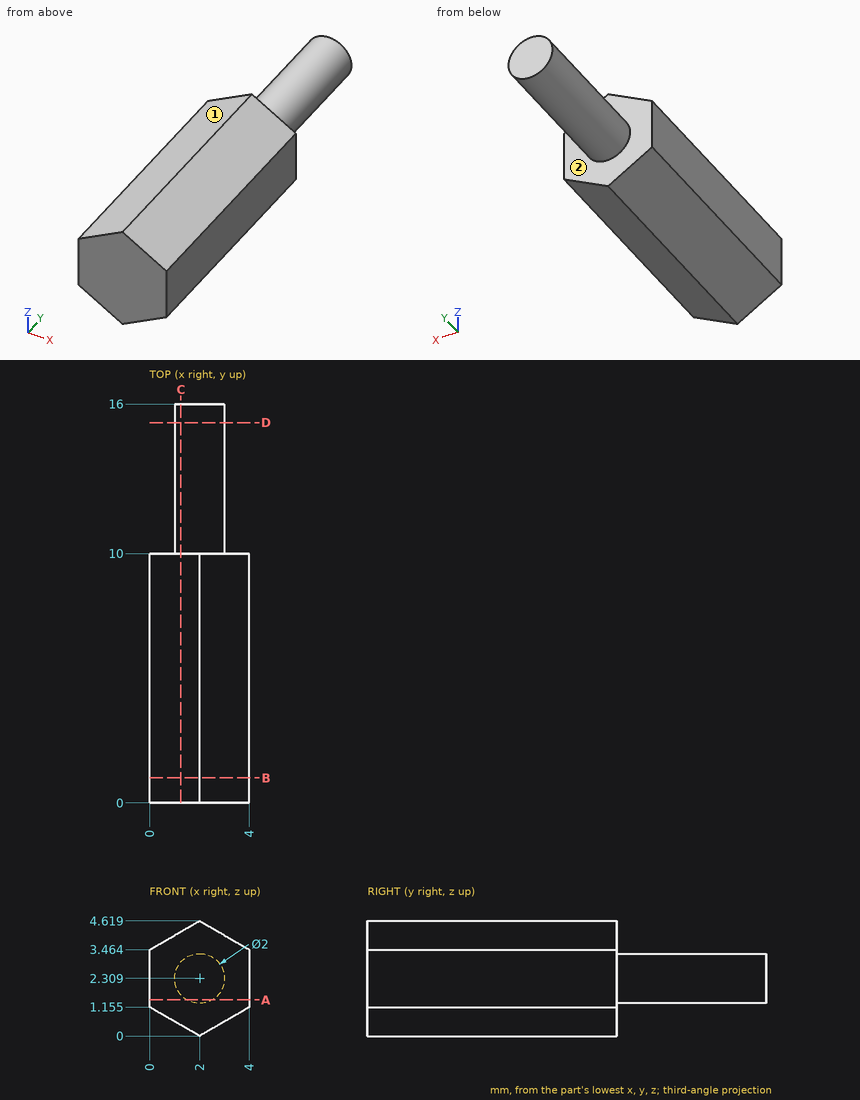
Geometry check sheet. Reference: drawing and pictorial views, mm from the part's lowest x, y, z. A direction names the side the tool comes from. Give positions to 0.01 mm unless a question says otherwise; leave off trailing zeros. Order: outer loops, then holes, each group sorted by start corner. A loop starts at its lowest first (then second) coordinate and runs counter-clockwise, first axis right, second up. Notation, with made-up numbers: M 73.5,46 L 102.5,46 A20 cw 102.5,68 Z; hole C -24,5.25 d8. An arc over 180 degrees is marked long. Answer in a Markdown table with one row per item. Add a question column.
Item 1: Section check C-C, the plane x = 1.25. Enter the section's corners in (y, z) (1 decimal).
Item 2: Section check B-B, the plane y = 1. Enter the section's corners in (x, z) (1 decimal).
Item 3: Scan lines: probe 1 along Y at (x, z) = (2.6, 1.2); probe 2 along Z at (x, y) = (2.75, 12.5); probe 3 along Z at (x, y) = (2.75, 6.75) (1 decimal). Record each from-to range of solid material in increasing order. Write a range as from..to.
Item 4: Section check D-D, the plane y = 15.25. Enter the section's corners in (x, z).
Item 5: Section check A-A, the plane z = 1.45. Enter the section's corners in (x, y).
Item 6: Tool access check on the marked faces 1 and 2. Record the directions out of +Z, -Z, +X, -X, +Y, -Y that give a thin tool (end or side, any length) a straight path to the whole face; none if there is none.
Item 7: Gauge pin test, flat end, axial feed: pin 1 (2 mm diameter, centred on x = 3.5, y = 8.5, fed in from +Z). Record the tip position at first contact, or that the pin passes through.
Filled sheet:
| question | item | result |
|---|---|---|
| 1 | outline | M 0,0.4 L 10,0.4 L 10,1.6 L 16,1.6 L 16,3 L 10,3 L 10,4.2 L 0,4.2 Z |
| 2 | outline | M 0,1.2 L 2,0 L 4,1.2 L 4,3.5 L 2,4.6 L 0,3.5 Z |
| 3 | probe 1 | y = 0..10 |
| 3 | probe 2 | z = 1.65..2.97 |
| 3 | probe 3 | z = 0.4..4.2 |
| 4 | outline | C 2,2.31 d2 |
| 5 | outline | M 0,0 L 4,0 L 4,10 L 2.51,10 L 2.51,16 L 1.49,16 L 1.49,10 L 0,10 Z |
| 6 | face 1 | +Z, -X, +Y, -Y |
| 6 | face 2 | +Y |
| 7 | pin 1 | stops at z = 4.33 |
